Geometry check sheet. Reference: the model listing, model coordinates, mm. A direction names the side the tool comes from. Coordinates: 2 decimals unless noted, no trailing zeros. Loops run counter-clockwise (first coordinate to the right, second up) from the corner with the lowest first, then second, coordinate; pieces in that order, holes last. Notation, with made-up numbers: (71, -17.5) - (87, -17.5) arc R22 cw to (87, 17.5) - close; hole circle Ø1 at (11.25, 66.5). An arc over 180 degrees is marked (long way). One line per item, written item: value.
from build123d import *

# Parameters (mm, degrees)
SKETCH1_R           = 65
SKETCH1_R_2         = 20
SKETCH1_R_3         = 3.25
BOSS_EXTRUDE1_DEPTH = 32
SKETCH2_R           = 55
SKETCH2_R_2         = 20
SKETCH2_R_3         = 2.6
BOSS_EXTRUDE2_DEPTH = 32
SKETCH3_W           = 100
SKETCH3_H           = 28
BOSS_EXTRUDE3_DEPTH = 24


with BuildPart() as part:
    # Sketch1 → Boss-Extrude1 (new body)
    with BuildSketch(Plane.XY):
        Circle(SKETCH1_R)
        Circle(SKETCH1_R_2, mode=Mode.SUBTRACT)
        with Locations((47.5, 0)):
            Circle(SKETCH1_R_3, mode=Mode.SUBTRACT)
        with Locations((23.75, 41.13620668)):
            Circle(SKETCH1_R_3, mode=Mode.SUBTRACT)
        with Locations((-23.75, 41.13620668)):
            Circle(SKETCH1_R_3, mode=Mode.SUBTRACT)
        with Locations((-47.5, 0)):
            Circle(SKETCH1_R_3, mode=Mode.SUBTRACT)
        with Locations((-23.75, -41.13620668)):
            Circle(SKETCH1_R_3, mode=Mode.SUBTRACT)
        with Locations((23.75, -41.13620668)):
            Circle(SKETCH1_R_3, mode=Mode.SUBTRACT)
    extrude(amount=BOSS_EXTRUDE1_DEPTH)



with BuildPart() as body_2:
    # Sketch2 → Boss-Extrude2 (new body)
    with BuildSketch(Plane.XY):
        with Locations((500, 0)):
            Circle(SKETCH2_R)
        with Locations((500, 0)):
            Circle(SKETCH2_R_2, mode=Mode.SUBTRACT)
        with Locations((476.43, -23.57)):
            Circle(SKETCH2_R_3, mode=Mode.SUBTRACT)
        with Locations((476.43, 23.57)):
            Circle(SKETCH2_R_3, mode=Mode.SUBTRACT)
        with Locations((523.57, -23.57)):
            Circle(SKETCH2_R_3, mode=Mode.SUBTRACT)
        with Locations((523.57, 23.57)):
            Circle(SKETCH2_R_3, mode=Mode.SUBTRACT)
    extrude(amount=BOSS_EXTRUDE2_DEPTH)


with BuildPart() as part_1:
    add(part.part)

    add(body_2.part)  # Boss-Extrude3 merges body 2
    # Sketch3 → Boss-Extrude3 (add)
    with BuildSketch(Plane.XY):
        Polygon((10, -35), (10, 35), (490, 27), (490, -27), align=None)
        with Locations((160, 0)):
            Rectangle(SKETCH3_W, SKETCH3_H, mode=Mode.SUBTRACT)
        with Locations((340, 0)):
            Rectangle(SKETCH3_W, SKETCH3_H, mode=Mode.SUBTRACT)
    extrude(amount=BOSS_EXTRUDE3_DEPTH)


solid = part_1.part
(1) Go/stop test with flat-tipped pins: pin 1 Ø3 at (x, y) = (12.5, -2) entering from +Z; pin 2 Ø6 at (y, z) = (29, 5) entering from -X; pin 3 Ø2 at (x, y) = (443, 22.5) entering from -Z; pin 4 Ø4 at (x, z) = (301.5, 10.5) entering from +Y (3 decimals). Record where each tip stops, or that it passes through.
Reply:
pin 1: z = 24
pin 2: x = -59.57
pin 3: z = 0
pin 4: y = 30.175
(2) Cross-section at B-B on y = 8.5. Record the cut outline in (x, z).
Reply:
outline: (-64.44, 0) - (-18.1, 0) - (-18.1, 32) - (-64.44, 32) - close; (10, 0) - (110, 0) - (110, 24) - (64.44, 24) - (64.44, 32) - (18.1, 32) - (18.1, 24) - (10, 24) - close; (210, 0) - (290, 0) - (290, 24) - (210, 24) - close; (390, 0) - (490, 0) - (490, 24) - (481.9, 24) - (481.9, 32) - (445.66, 32) - (445.66, 24) - (390, 24) - close; (518.1, 0) - (554.34, 0) - (554.34, 32) - (518.1, 32) - close
(3) Release check for a two-part mould opening along Y. For faces 4 (the face through (257, 0, 24)), 5 (the face through (550.806, -21.065, 15.776)), 6 (the face through (339, 14, 12)) record: pulls with the +Y half, pulls with the -Y half, needs draft (parallel to the pull), parting line crosses it, or undercut.
Reply:
face 4: needs draft
face 5: parting line crosses it
face 6: undercut
(4) Cross-section at C-C on x = 0. Record the cut outline in (y, z).
Reply:
outline: (-65, 0) - (-20, 0) - (-20, 32) - (-65, 32) - close; (20, 0) - (65, 0) - (65, 32) - (20, 32) - close
(5) Cross-section at A-A on x = 500. Record the cut outline in (y, z).
Reply:
outline: (-55, 0) - (-20, 0) - (-20, 32) - (-55, 32) - close; (20, 0) - (55, 0) - (55, 32) - (20, 32) - close
(6) Cross-section at D-D on z = 8. State how many separate pieces and enclosed holes the cut face has, and give its area (3 significant figures).
Reply:
separate pieces: 1
enclosed holes: 11
area: 38,800 mm2
(7) Material ranges on probe 1 along Y at (x, z) = (-23.75, 13); probe 2 along X at (y, z) = (23, 26); probe 3 along Y at (x, z) = (523.57, 10.5), recorded low to high. Write a range as from..to.
Reply:
probe 1: -60.51..-44.39, -37.89..37.89, 44.39..60.51
probe 2: -60.79..60.79, 450.04..473.89, 478.97..521.03, 526.11..549.96
probe 3: -49.69..-26.17, -20.97..20.97, 26.17..49.69
(8) Access from +Z, -Z, +X, -X, +Y, -Y to the whole of each face (thin tool, end or side, straight path). Record for faces 1 (the face through (524, 1, 32)), 2 (the face through (390, 0, 12)), 3 (the face through (14, 0, 24)).
Reply:
face 1: +Z, +X, -X, +Y, -Y
face 2: +Z, -Z
face 3: +Z
